Could you check a few things on this model? Use its own coordinates, in mm. Face numbers are marked on the shaded views. Round coordinates to 2 decimals unless told otherwise and drop trailing zeros. Loops run counter-clockwise (first coordinate to the right, second up) from the corner with the lowest first, then second, coordinate; pieces in that order, holes last. Notation, with made-up numbers: (76.5, 58) -> (122.5, 58) arc R9 cw to (122.5, 73) -> close; hole circle Ø9 at (29.5, 29). An arc over 180 degrees is marked (long way). Put each result on its own line as item: value. Start each with the question number.
1. Imagine slicing it at B-B, the plane y = 29. Please give me the cut outline in (x, z), and give its area (3 significant figures).
2. Imagine slicing it at A-A, the plane z = 5.05. Please give me the cut outline in (x, y).
3. If we mould it in two halves opening along X, with no side actions, what happens to the marked faces 1, 2, 3 and 4? For each: pulls with the +X half, pulls with the -X half, needs draft (parallel to the pull), parting line crosses it, or undercut.
4. I need wall thicknesses on line 1 (Y direction, x = -4.75, z = 5.75); line 2 (X direction, y = -29.5, z = 5.1); line 3 (Z direction, x = -4.75, y = 56.5). Which ranges of each line are inside material? Lowest first, please. Write a range as [from, to].
5. I'm going to push flat-ended pins straight in: P1, Ø6, axis at x = 0.5, y = -5, coming from the +Z side; P2, Ø1.5, axis at x = -9, y = 2.5, coming from the -Z side. Where does each tip first touch, or does it pass through?
6. Imagine slicing it at C-C, the plane x = -4.5. Please give me the cut outline in (y, z).
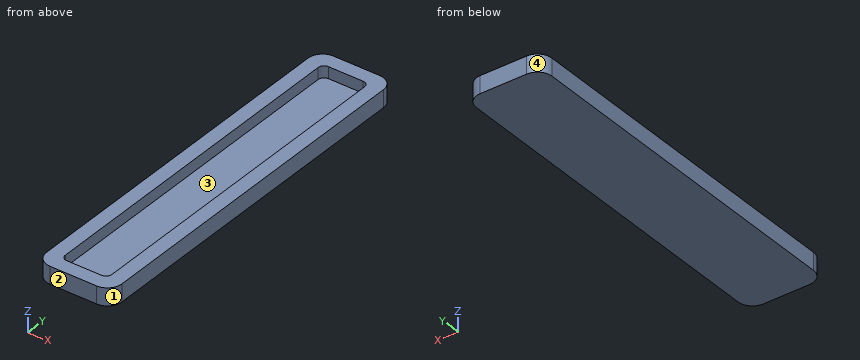
```python
from build123d import *

# Parameters (mm, degrees)
F0_W     = 26
F0_H     = 130
F1_DEPTH = 6
F2_W     = 16
F2_H     = 120
F3_DEPTH = 4
F4_R     = 2
F5_R     = 5


with BuildPart() as f1:
    # F0 (on Top) → F1 (new body)
    with BuildSketch(Plane.XY):
        Rectangle(F0_W, F0_H)
    extrude(amount=F1_DEPTH)

    # F2 (on face) → F3 (cut)
    with BuildSketch(Plane.XY.offset(6)):
        Rectangle(F2_W, F2_H)
    extrude(amount=-F3_DEPTH, mode=Mode.SUBTRACT)

    # F4
    f4_edges = [f1.edges().sort_by_distance(p)[0] for p in [
        (-8, 60, 4),
        (-8, -60, 4),
        (8, -60, 4),
        (8, 60, 4),
    ]]
    fillet(f4_edges, radius=F4_R)

    # F5
    f5_edges = [f1.edges().sort_by_distance(p)[0] for p in [
        (-13, -65, 3),
        (13, -65, 3),
        (13, 65, 3),
        (-13, 65, 3),
    ]]
    fillet(f5_edges, radius=F5_R)


solid = f1.part
```
Entries:
1. outline: (-13, 0) -> (13, 0) -> (13, 6) -> (8, 6) -> (8, 2) -> (-8, 2) -> (-8, 6) -> (-13, 6) -> close
1. area: 92.0 mm^2
2. outline: (-13, -60) arc R5 ccw to (-8, -65) -> (8, -65) arc R5 ccw to (13, -60) -> (13, 60) arc R5 ccw to (8, 65) -> (-8, 65) arc R5 ccw to (-13, 60) -> close; hole (-8, -58) arc R2 ccw to (-6, -60) -> (6, -60) arc R2 ccw to (8, -58) -> (8, 58) arc R2 ccw to (6, 60) -> (-6, 60) arc R2 ccw to (-8, 58) -> close
3. face 1: pulls with the +X half
3. face 2: needs draft
3. face 3: undercut
3. face 4: pulls with the -X half
4. line 1: [-65, -60], [60, 65]
4. line 2: [-13, -8], [8, 13]
4. line 3: [0, 2]
5. P1: z = 2
5. P2: z = 0
6. outline: (-65, 0) -> (65, 0) -> (65, 6) -> (60, 6) -> (60, 2) -> (-60, 2) -> (-60, 6) -> (-65, 6) -> close
